from build123d import *

# Parameters (mm, degrees)
SKETCH1_W           = 87.8
SKETCH1_H           = 87.8
BOSS_EXTRUDE1_DEPTH = 2
SKETCH1_3_W         = 87.8
SKETCH1_3_H         = 87.8
SKETCH1_3_W_2       = 83
SKETCH1_3_H_2       = 83
BOSS_EXTRUDE2_DEPTH = 20
SKETCH2_OUTSIDE_W   = 115.02
SKETCH2_OUTSIDE_H   = 115.02
SKETCH2_OUTSIDE_W_2 = 84.6
SKETCH2_OUTSIDE_H_2 = 84.6
CUT_EXTRUDE1_DEPTH  = 1.4


with BuildPart() as part:
    # Sketch1 → Boss-Extrude1 (new body)
    with BuildSketch(Plane.XY):
        with Locations((41.5, 41.5)):
            Rectangle(SKETCH1_W, SKETCH1_H)
    extrude(amount=-BOSS_EXTRUDE1_DEPTH)

    # Sketch1<3> → Boss-Extrude2 (add)
    with BuildSketch(Plane.XY):
        with Locations((41.5, 41.5)):
            Rectangle(SKETCH1_3_W, SKETCH1_3_H)
        with Locations((41.5, 41.5)):
            Rectangle(SKETCH1_3_W_2, SKETCH1_3_H_2, mode=Mode.SUBTRACT)
    extrude(amount=BOSS_EXTRUDE2_DEPTH)

    # Sketch2 outside → Cut-Extrude1 (cut)
    with BuildSketch(Plane.XY.offset(20)):
        with Locations((41.5, 41.5)):
            Rectangle(SKETCH2_OUTSIDE_W, SKETCH2_OUTSIDE_H)
        with Locations((41.5, 41.5)):
            Rectangle(SKETCH2_OUTSIDE_W_2, SKETCH2_OUTSIDE_H_2, mode=Mode.SUBTRACT)
    extrude(amount=-CUT_EXTRUDE1_DEPTH, mode=Mode.SUBTRACT)


solid = part.part
Design review of the part built by this model. Coordinates are the model's own, in mm. A direction names the side the tool comes from. Coordinates: 2 decimals unless noted, no trailing zeros. Order: outer loops, then holes, each group sorted by start corner. A loop starts at its lowest first (then second) coordinate and runs counter-clockwise, first axis right, second up. Notation, with made-up numbers: (30.25, 18.25) - (89.25, 18.25) arc R9 cw to (89.25, 33.25) - close; hole circle Ø7 at (-3, 40). An arc over 180 degrees is marked (long way). Put each result on its own line as item: value.
1) Tool access review of faces 4 (the face through (41, 42, 0)), 5 (the face through (85.4, 41, 8)): name each direction out of +Z, -Z, +X, -X, +Y, -Y from which nothing blocks a thin tool from reaching the whole face with its end or side.
Response values:
face 4: +Z
face 5: +Z, -Z, +X, +Y, -Y
2) Take a section at B-B, the plane y = 38. Give the boundary of the cut face in (x, z).
Response values:
outline: (-2.4, -2) - (85.4, -2) - (85.4, 18.6) - (83.8, 18.6) - (83.8, 20) - (83, 20) - (83, 0) - (0, 0) - (0, 20) - (-0.8, 20) - (-0.8, 18.6) - (-2.4, 18.6) - close
3) Wall thickness on L1, parallel to X at y = 17, z = 6; L2, parallel to Y at x = 57, z = 19.25: over which ranges is each line inside the solid? List them lowest first. Write a range as from..to.
Response values:
L1: x = -2.4..0, 83..85.4
L2: y = -0.8..0, 83..83.8
4) Take a section at A-A, the plane z = 2.75. Give the boundary of the cut face in (x, y).
Response values:
outline: (-2.4, -2.4) - (85.4, -2.4) - (85.4, 85.4) - (-2.4, 85.4) - close; hole (0, 0) - (83, 0) - (83, 83) - (0, 83) - close
5) Insertion check: P1, Ø1.5, axis at x = 23, y = 18, coming from the +Z side; P2, Ø1.5, axis at x = 47.5, z = 19.5, coming from the -Y side; P3, Ø1.5, axis at x = 36, z = 19.5, coming from the +Y side. Each pin has a flat end and moves straight along its axis. Give the tip position at first contact, or say it passes through.
Response values:
P1: stops at z = 0
P2: stops at y = -0.8
P3: stops at y = 83.8
6) The part is to be moulded in two halves that separate along Y. For faces 1 (the face through (-2.4, 41, 8)), 2 (the face through (0, 41, 10)), 3 (the face through (41, 85.4, 8)), say which applies: released by +Y, released by -Y, zero draft, split by the parting line, or undercut.
Response values:
face 1: zero draft
face 2: undercut
face 3: released by +Y
